Part print with two shaded views. Sizes in mm from the minimum x, y, z corner. A direction names the side the tool comes from. Give positions to 0.01 mm unless a question says otherwise; leave off trailing zeros. Write each loop counter-clockwise with the first axis right and the second up, starting at its lowest first coordinate (ties: lowest second). Pieces come first, ordered by that corner, then holes.
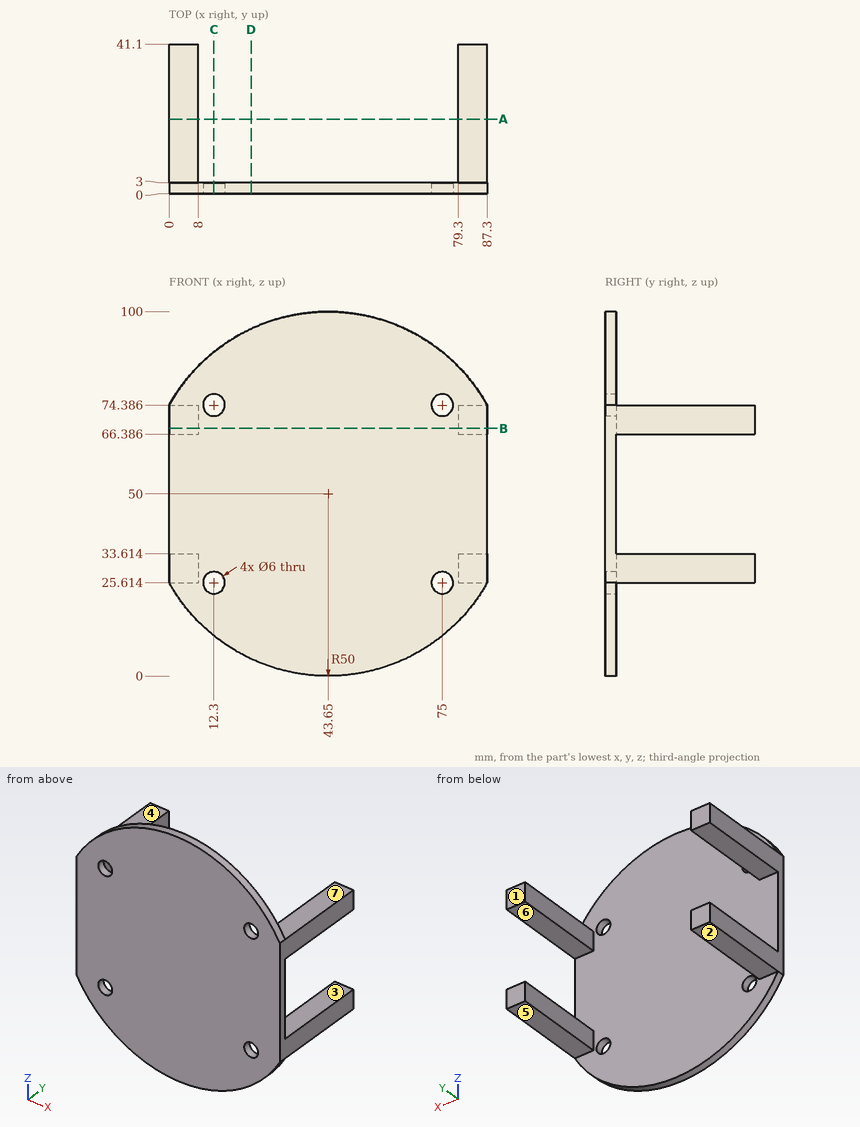
(1) Mould opens along Z. For the marked faces 5, 6 and 7 say: +Z half, -Z half, draft (parallel to the pull), parting line (faces both ways), or undercut.
(2) Saw through at C-C, the plane x = 12.3. List the corners of the cut face in (y, z).
(3) Saw through at D-D, the plane x = 22.5. List the corners of the cut face in (y, z).
(4) Probe line 1 (Z direction, x = 4.5, y = 13); line 2 (Z direction, x = 12, y = 1); line 3 (Y direction, x = 22, z = 17.5). List the from-to ranges inside material, lowest first.
(5) Saw through at A-A, the plane y = 20.5. List the corners of the cut face in (x, z).
(6) Drop flat-ended pins along their axis: pin 1 (9 mm diameter, centred on x = 82, y = 13.5, fed in from +Z); pin 2 (9 mm diameter, centred on x = 4, y = 12.5, fed in from -Z); pin 3 (7 mm diameter, centred on x = 75, z = 74.39, fed in from +Y). Give the stop position or say it passes through.
(7) Saw through at B-B, the plane z = 68. List the corners of the cut face in (x, y).
(8) 3-axis set-ups, long thin cutter, end or side, ignore diameter. For the marked faces 1, 2, 3 and 4: which of +Z, -Z, +X, -X, +Y, -Y reach the whole face in a straight line?
Computed values:
1. face 5: -Z half
1. face 6: undercut
1. face 7: +Z half
2. outline: (0, 11.05) - (3, 11.05) - (3, 22.61) - (0, 22.61) - close; (0, 28.61) - (3, 28.61) - (3, 71.39) - (0, 71.39) - close; (0, 77.39) - (3, 77.39) - (3, 88.95) - (0, 88.95) - close
3. outline: (0, 4.69) - (3, 4.69) - (3, 95.31) - (0, 95.31) - close
4. line 1: z = 25.61 to 33.61, 66.39 to 74.39
4. line 2: z = 11.29 to 22.63, 28.6 to 71.4, 77.37 to 88.71
4. line 3: y = 0 to 3
5. outline: (0, 25.61) - (8, 25.61) - (8, 33.61) - (0, 33.61) - close; (0, 66.39) - (8, 66.39) - (8, 74.39) - (0, 74.39) - close; (79.3, 25.61) - (87.3, 25.61) - (87.3, 33.61) - (79.3, 33.61) - close; (79.3, 66.39) - (87.3, 66.39) - (87.3, 74.39) - (79.3, 74.39) - close
6. pin 1: stops at z = 74.39
6. pin 2: stops at z = 25.61
6. pin 3: stops at y = 3
7. outline: (0, 0) - (87.3, 0) - (87.3, 41.1) - (79.3, 41.1) - (79.3, 3) - (8, 3) - (8, 41.1) - (0, 41.1) - close
8. face 1: +Z, -Z, +X, -X, +Y
8. face 2: -Z, +X, -X, +Y
8. face 3: +X, -X, +Y
8. face 4: +Z, +X, -X, +Y
